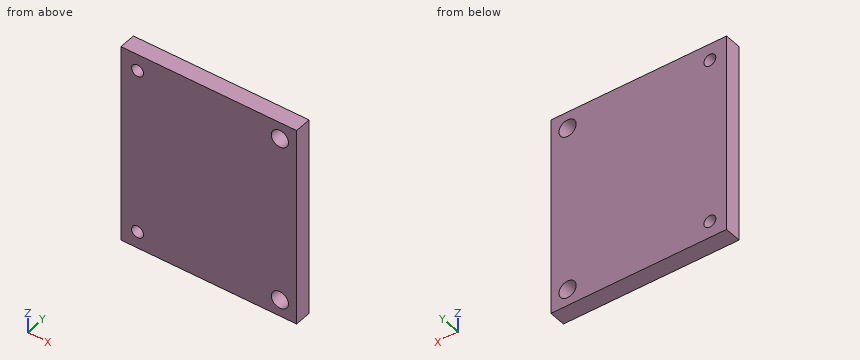
from build123d import *

# Parameters (mm, degrees)
F0_W     = 73.7
F0_H     = 84
F0_R     = 2.5
F0_R_2   = 3.6
F1_DEPTH = 7


with BuildPart() as f1:
    # F0 (on Front) → F1 (new body)
    with BuildSketch(Plane.XZ):
        with Locations((-32.094777, 21.537357)):
            Rectangle(F0_W, F0_H)
        with Locations((-61.944777, -13.462643)):
            Circle(F0_R, mode=Mode.SUBTRACT)
        with Locations((-2.244777, -13.462643)):
            Circle(F0_R_2, mode=Mode.SUBTRACT)
        with Locations((-61.944777, 56.537357)):
            Circle(F0_R, mode=Mode.SUBTRACT)
        with Locations((-2.244777, 56.537357)):
            Circle(F0_R_2, mode=Mode.SUBTRACT)
    extrude(amount=F1_DEPTH)


solid = f1.part
Can you work these out from the model? Positions are in its coordinate system, mm. Coordinates: 2 decimals unless noted, no trailing zeros. Loops run counter-clockwise (first coordinate to the right, second up) from the corner with the lowest first, then second, coordinate; pieces in that order, holes last. Notation, with made-up numbers: M -29,88.25 L -16,88.25 A26 cw -16,109.25 Z; hole C 44.5,65.5 d1. An arc over 180 degrees is marked long. Answer as CSV lines item,"result". Start each with the question number.
1. For pin 1 Ø3 at (x, z) = (-61.94, 56.54) entering from -Y, with a flat end and sliding along its axis, tell me the tip position at first contact or that it passes through.
2. If I drill on probe 1 along Z at (x, y) = (-5.5, -2); probe 2 along X at (y, z) = (-3, -15); probe 3 along X at (y, z) = (-4.5, 59.5), over which ranges is the centre line in solid material (lowest first)? Write a range as [from, to].
3. Suppose I cut it at B-B, the plane x = -1. List the corners of the cut face in (y, z) for me.
4. Suppose I cut it at A-A, the plane y = -3.5. List the corners of the cut face in (x, z) for me.
Output:
1,pin 1,"passes through"
2,probe 1,"z = [-20.46, -15], [-11.93, 55], [58.07, 63.54]"
2,probe 2,"x = [-68.94, -63.92], [-59.97, -5.5], [1.01, 4.76]"
2,probe 3,"x = [-68.94, -4.29], [-0.2, 4.76]"
3,outline,"M -7,-20.46 L 0,-20.46 L 0,-16.84 L -7,-16.84 Z; M -7,-10.08 L 0,-10.08 L 0,53.16 L -7,53.16 Z; M -7,59.92 L 0,59.92 L 0,63.54 L -7,63.54 Z"
4,outline,"M -68.94,-20.46 L 4.76,-20.46 L 4.76,63.54 L -68.94,63.54 Z; hole C -61.94,-13.46 d5; hole C -61.94,56.54 d5; hole C -2.24,-13.46 d7.2; hole C -2.24,56.54 d7.2"
